```python
from build123d import *

# Parameters (mm, degrees)
F1_DEPTH = 1219.2
F3_DEPTH = 127


with BuildPart() as f1:
    # F0 (on Front) → F1 (new body)
    with BuildSketch(Plane.XZ):
        Polygon((30.604916, -12.676971), (30.604916, 12.676971), (12.676971, 30.604916), (-12.676971, 30.604916), (-30.604916, 12.676971), (-30.604916, -12.676971), (-12.676971, -30.604916), (12.676971, -30.604916), align=None)
    extrude(amount=F1_DEPTH)

    # F2 (on face) → F3 (join)
    with BuildSketch(Plane(origin=(-30.604916, 0, 0), x_dir=(0, -1, 0), z_dir=(-1, 0, 0))):
        Polygon((581.44556, 12.676971), (637.815356, 12.676971), (633.938922, 22.903467), (610.61502, 33.405414), (586.696533, 24.338922), align=None)
        Polygon((637.75444, -12.676971), (643.005414, -1.01502), (637.815356, 12.676971), (581.44556, 12.676971), (576.194586, 1.01502), (581.384644, -12.676971), align=None)
        Polygon((632.503467, -24.338922), (637.75444, -12.676971), (581.384644, -12.676971), (585.261078, -22.903467), (608.58498, -33.405414), align=None)
    extrude(amount=F3_DEPTH)


solid = f1.part
```
The listing builds one solid part. Answer for the finished solid, in the listing's coordinates (mm). A direction names the side the tool comes from. Round coordinates to 2 decimals unless told otherwise and drop trailing zeros. Loops run counter-clockwise (first coordinate to the right, second up) from the corner with the lowest first, then second, coordinate; pieces in that order, holes last.
1) For faces 1 (the face through (-93.216, -598.823, 28.936)), 2 (the face through (-30.605, -287, 0)), 3 (the face through (-93.2, -622.4, 28.1)), 4 (the face through (-93.216, -620.377, -28.936)), determine the directions among +Z, -Z, +X, -X, +Y, -Y from which every point of the face is accessible in a straight line to the end or side of a thin tool.
Outcome:
face 1: +Z, -X, +Y
face 2: +Z, -Z, -X, +Y
face 3: +Z, -X, -Y
face 4: -Z, -X, -Y
2) Consider line 1 (Z direction, x = 5, y = -528); line 2 (Z direction, x = -61, y = -611). Determine where each line is inside the solid, lowest interval first.
Outcome:
line 1: z = -30.6 to 30.6
line 2: z = -32.49 to 33.23
3) A cutting plane is placed at B-B on y = -386.5. Determine the outline of the cut face in (x, z).
Outcome:
outline: (-30.6, -12.68) - (-12.68, -30.6) - (12.68, -30.6) - (30.6, -12.68) - (30.6, 12.68) - (12.68, 30.6) - (-12.68, 30.6) - (-30.6, 12.68) - close
4) A cutting plane is placed at A-A on x = -113.5. Determine the outline of the cut face in (y, z), plus the area to 3 significant figures.
Outcome:
outline: (-643.01, -1.02) - (-632.5, -24.34) - (-608.58, -33.41) - (-585.26, -22.9) - (-576.19, 1.02) - (-586.7, 24.34) - (-610.62, 33.41) - (-633.94, 22.9) - close
area: 3,160 mm2
5) Given P1, Ø4, axis at y = -740.5, z = -24.5, coming from the -X side; P2, Ø7.5, axis at y = -824.5, z = -4, coming from the -X side; P3, Ø2, axis at x = -70, z = 16, coming from the -Y side, each flat-ended and moving along its own axis, determine where each tip first touches the part or whether it passes through.
Outcome:
P1: stops at x = -20.78
P2: stops at x = -30.6
P3: stops at y = -636.93
